Input: part model. Units: mm. Frame: model coordinates. A direction names the side the tool comes from. Coordinates: 2 decimals unless noted, no trailing zeros. Loops run counter-clockwise (first coordinate to the right, second up) from the corner with the lowest first, then second, coordinate; pieces in that order, holes last. Notation, with made-up numbers: (-22, -5) -> (34, -5) arc R14 ccw to (34, 19) -> close; hole circle Ø2 at (-33, 88). An arc over 180 degrees is marked (long way). Put each result on its own line as item: value. Start each with the question number.
1) Cut plane C-C (y = 1.25). State how many separate pieces and enclosed holes the cut face has, plus the area to 3 significant figures.
2) Set-up query: faces 1 (the flat face through (-1, 3, 57.15)), 2 (the flat face through (-57.15, 3, 16)). Return all of +Z, -Z, +X, -X, +Y, -Y with unobstructed straight access to the full face (end or side cutting, diameter ignored); none if empty.
3) Pull-direction query (X, two-part tool) for faces 3 (the cylindrical face through (-59.69, 3.13, -13.84)), 4 (the cylindrical face through (-15.497, 3.219, 16.991)), 5 (the cylindrical face through (59.82, 3.13, -13.97)); classes: pulls with the +X half, pulls with the -X half, needs draft (parallel to the pull), parting line crosses it, or undercut.
4) Cut plane D-D (z = 6.5). Return the cut outline in (x, y), plus the area to 3 significant figures.
5) Contact query for flat-ended pins moving along their axis: P1, Ø1.9, axis at y = 3, z = 9, coming from the -X side; P2, Ø2, axis at x = -67, y = 3.5, coming from the +Z side; P3, Ø3, axis at y = 3, z = 26.5, coming from the +X side; P4, Ø5, axis at x = -63.5, z = -44.45, coming from the -Y side. Output: stop coordinate, or through.
6) Cut plane A-A (z = -44.45). Return the cut outline in (x, y).
7) Material intervals for L1, parallel to Z at x = -17.5, y = 3.75; L2, parallel to Z at x = 18, y = 2; L3, parallel to X at y = 4, z = 37, sorted ascending.
8) Cut plane B-B (x = 12.5). Return the cut outline in (y, z), plus the area to 3 significant figures.
from build123d import *

# Parameters (mm, degrees)
SKETCH1_W           = 114.3
SKETCH1_H           = 114.3
BOSS_EXTRUDE1_DEPTH = 6.35
SKETCH3_W           = 19.05
SKETCH3_H           = 40.64
BOSS_EXTRUDE2_DEPTH = 6.35
SKETCH2_R           = 4.064
SKETCH2_R_2         = 17.4625
SKETCH2_R_3         = 2.286
CUT_EXTRUDE1_DEPTH  = 7.35
FILLET1_R           = 8.89
FILLET2_R           = 17.78
FILLET3_R           = 7.62


with BuildPart() as part:
    # Sketch1 → Boss-Extrude1 (new body)
    with BuildSketch(Plane(origin=(0, 0, 0), x_dir=(1, 0, 0), z_dir=(0, 1, 0))):
        Rectangle(SKETCH1_W, SKETCH1_H)
    extrude(amount=BOSS_EXTRUDE1_DEPTH)

    # Sketch3 → Boss-Extrude2 (add)
    with BuildSketch(Plane(origin=(0, 6.35, 0), x_dir=(1, 0, 0), z_dir=(0, 1, 0))):
        with Locations((66.675, 36.83)):
            Rectangle(SKETCH3_W, SKETCH3_H)
        with Locations((-66.675, 36.83)):
            Rectangle(SKETCH3_W, SKETCH3_H)
    extrude(amount=-BOSS_EXTRUDE2_DEPTH)

    # Sketch2 → Cut-Extrude1 (cut, through all)
    with BuildSketch(Plane(origin=(0, 6.35, 0), x_dir=(1, 0, 0), z_dir=(0, 1, 0))):
        with Locations((-63.5, 44.45)):
            Circle(SKETCH2_R)
        with Locations((63.5, 44.45)):
            Circle(SKETCH2_R)
        with Locations((44.45, -38.1)):
            Circle(SKETCH2_R)
        with Locations((-44.45, -38.1)):
            Circle(SKETCH2_R)
        Circle(SKETCH2_R_2)
        with Locations((-17.67766953, 17.67766953)):
            Circle(SKETCH2_R_3)
        with Locations((17.67766953, 17.67766953)):
            Circle(SKETCH2_R_3)
        with Locations((17.67766953, -17.67766953)):
            Circle(SKETCH2_R_3)
        with Locations((-17.67766953, -17.67766953)):
            Circle(SKETCH2_R_3)
    extrude(amount=-CUT_EXTRUDE1_DEPTH, mode=Mode.SUBTRACT)

    # Fillet1
    fillet1_edges = [part.edges().sort_by_distance(p)[0] for p in [
        (57.15, 3.175, -16.51),
        (-57.15, 3.175, -16.51),
    ]]
    fillet(fillet1_edges, radius=FILLET1_R)

    # Fillet2
    fillet2_edges = [part.edges().sort_by_distance(p)[0] for p in [
        (57.15, 3.175, 57.15),
        (-57.15, 3.175, 57.15),
    ]]
    fillet(fillet2_edges, radius=FILLET2_R)

    # Fillet3
    fillet3_edges = [part.edges().sort_by_distance(p)[0] for p in [
        (76.2, 3.175, -16.51),
        (76.2, 3.175, -57.15),
        (-76.2, 3.175, -57.15),
        (-76.2, 3.175, -16.51),
    ]]
    fillet(fillet3_edges, radius=FILLET3_R)


solid = part.part
Results found:
1. separate pieces: 1
1. enclosed holes: 9
1. area: 13,200 mm2
2. face 1: +Z, +X, -X, +Y, -Y
2. face 2: +Z, -X, +Y, -Y
3. face 3: pulls with the -X half
3. face 4: undercut
3. face 5: pulls with the +X half
4. outline: (-57.15, 0) -> (-16.21, 0) -> (-16.21, 6.35) -> (-57.15, 6.35) -> close; (16.21, 0) -> (57.15, 0) -> (57.15, 6.35) -> (16.21, 6.35) -> close
4. area: 520 mm2
5. P1: stops at x = -57.15
5. P2: stops at z = -16.51
5. P3: stops at x = 57.15
5. P4: passes through
6. outline: (-76.2, 0) -> (-67.56, 0) -> (-67.56, 6.35) -> (-76.2, 6.35) -> close; (-59.44, 0) -> (59.44, 0) -> (59.44, 6.35) -> (-59.44, 6.35) -> close; (67.56, 0) -> (76.2, 0) -> (76.2, 6.35) -> (67.56, 6.35) -> close
7. L1: z = -57.15 to -19.96, -15.4 to 15.4, 19.96 to 57.15
7. L2: z = -57.15 to -19.94, -15.41 to 15.41, 19.94 to 57.15
7. L3: x = -57.15 to -48.36, -40.54 to 40.54, 48.36 to 57.15
8. outline: (0, -57.15) -> (6.35, -57.15) -> (6.35, -12.19) -> (0, -12.19) -> close; (0, 12.19) -> (6.35, 12.19) -> (6.35, 57.15) -> (0, 57.15) -> close
8. area: 571 mm2
